Autodesk Fusion 360 part; units mm, degrees
sketch "Sketch1" plane through (0, 0, 0) normal (0, 1, 0) x (1, 0, 0)
  circle A0 centre (0, 0) radius 11
  circle A1 centre (0, 0) radius 12.5
  line L0 (0, 0) -> (9.5756, 8.0348)
  line L1 (0, 0) -> (12.5, 0) construction
  line L2 (0, 0) -> (-9.5756, 8.0348)
  line L3 (0, 0) -> (12.5, 0) construction
  line L4 (0, 0) -> (-4.7878, 11.5467)
  line L5 (-4.7878, 11.5467) -> (4.7878, 11.5467)
  circle A2 centre (0, 11.5467) radius 4.8552
  line L6 (0, 11.5467) -> (0, 16.402)
  circle A3 centre (0, 13.9744) radius 1.05
  circle A4 centre (0, 13.9744) radius 0.5
  line L7 (0, 16.402) -> (-0.6, 16.402)
  line L8 (0, 16.402) -> (0.6, 16.402)
  line L9 (-0.6, 16.402) -> (-0.6, 14.836)
  line L10 (0.6, 16.402) -> (0.6, 14.836)
  line L11 (0, 0) -> (6.25, 10.8253)
  line L12 (0, 0) -> (12.5, 0) construction
  line L13 (0, 0) -> (-6.25, 10.8253)
  line L14 (0, 11.5467) -> (2, 11.5467)
  line L15 (0, 11.5467) -> (-2, 11.5467)
  line L16 (2, 11.5467) -> (-2, 11.5467)
  line L17 (-2, 11.5467) -> (-2, 15.9709)
  line L18 (-2, 15.9709) -> (2, 15.9709)
  line L19 (2, 15.9709) -> (2, 11.5467)
  dimension "d1" = 22
  dimension "d2" = 25
  dimension "d3" = 40
  dimension "d4" = 140
  dimension "d5" = 2.1
  dimension "d6" = 1
  dimension "d7" = 0.6
  dimension "d8" = 0.6
  dimension "d9" = 60
  dimension "d10" = 120
  dimension "d13" = 2
  dimension "d14" = 2
  dimension "d15" = 9.5756
  dimension "d16" = 4.4242
extrude "Extrude1" add sketch "Sketch1" along normal blind 12 contours A0 A1 A2 L11 | A0 A1 A2 L13 | A0 A1 L4 L5 A2 L14 L15 L16 | A0 A1 L4 A2 | A1 L5 L17 | A1 L5 L19 | A1 L6 A3 L9 L17 L18 | A2 L9 L18 | A1 L5 L6 L15 L16 L17 | A1 L5 L6 L14 L16 L19 | A1 L6 A3 L10 L18 L19 | A2 L10 L18
sketch "Sketch2" plane through (0, 0, 0) normal (0, -1, 0) x (1, 0, 0)
  line L0 (0.6, -14.836) -> (0.6, -16.3648)
  arc A0 (0.6, -16.3648) -> (2, -15.9709) centre (0, -11.5467) ccw
  line L1 (2, -15.9709) -> (2, -12.339)
  arc A1 (2, -12.339) -> (6.25, -10.8253) centre (0, 0) ccw
  line L2 (6.25, -10.8253) -> (5.5, -9.5263)
  arc A2 (-5.5, -9.5263) -> (5.5, -9.5263) centre (0, 0) ccw
  line L3 (-5.5, -9.5263) -> (-6.25, -10.8253)
  arc A3 (-6.25, -10.8253) -> (-2, -12.339) centre (0, 0) ccw
  line L4 (-2, -12.339) -> (-2, -15.9709)
  arc A4 (-2, -15.9709) -> (-0.6, -16.3648) centre (0, -11.5467) ccw
  line L5 (-0.6, -16.3648) -> (-0.6, -14.836)
  arc A5 (0.6, -14.836) -> (-0.6, -14.836) centre (0, -13.9744) ccw
  line L6 (0, -11) -> (0, -12.9244)
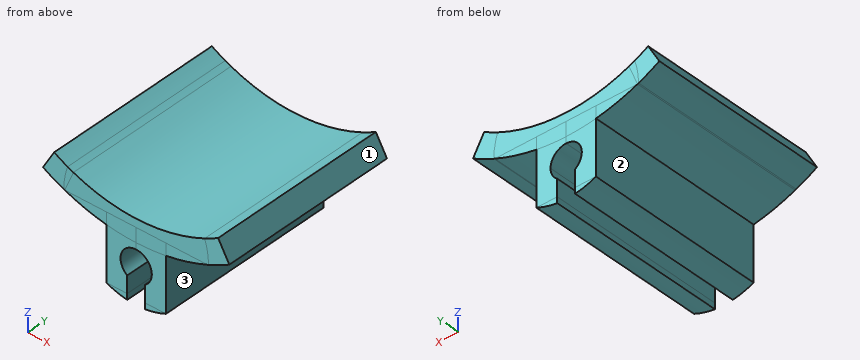
Verification items for the finished model (mm, model axes). Face numbers are marked on the shaded views. A direction names the side the tool comes from. Coordinates: 2 decimals unless noted, no trailing zeros. Write each loop counter-clockwise with the first axis right and the second up, starting at its lowest first coordinate (ties: lowest second). Pieces come first, ordered by that corner, then holes. Notation, with made-up numbers: M 49.25,60 L 103.25,60 A29 cw 103.25,93 Z; hole C 37,-18.75 d7. An arc over 180 degrees is marked long. One line per item, written item: value.
Item 1: Gauge pin test, flat ends, axial feed: pin 1 Ø1.1 at (y, z) = (5, -14.5) entering from -X; pin 2 Ø3 at (y, z) = (3, -14.5) entering from +X; pin 3 Ø3 at (x, y) = (3.5, 6.5) entering from +Z. Record the tip position at first contact, or that the pin passes through.
Check sheet entries:
pin 1: stops at x = -2
pin 2: stops at x = 2
pin 3: stops at z = -9.8
Item 2: Section check D-D, the plane x = -1.5. Record the boundary of the cut face in (y, z), plus the area to 3 significant figures.
Check sheet entries:
outline: M 0,-16.16 L 12,-16.16 L 12,-10.9 L 0,-10.9 Z
area: 63.2 mm^2
Item 3: Scan lines: line 1 along X through (y, z) = (11.25, -14); line 2 along X through (y, z) = (1, -15.75); line 3 along Z through (x, y) = (1.75, 8.75). Record each from-to range of solid material in increasing order.
Check sheet entries:
line 1: x = -2 to -1.05, 1.05 to 2
line 2: x = -2 to -0.6, 0.6 to 2
line 3: z = -16.08 to -10.86
Item 4: Section check A-A, the plane z = -15.25. Record the boundary of the cut face in (x, y), plus the area to 3 significant figures.
Check sheet entries:
outline: M -2,0 L -0.6,0 L -0.6,12 L -2,12 Z; M 0.6,0 L 2,0 L 2,12 L 0.6,12 Z
area: 33.6 mm^2
Item 5: Section check C-C, the plane z = -13.5. Record the boundary of the cut face in (x, y), plus the area to 3 significant figures.
Check sheet entries:
outline: M -2,0 L -0.94,0 L -0.94,12 L -2,12 Z; M 0.94,0 L 2,0 L 2,12 L 0.94,12 Z
area: 25.5 mm^2
Item 6: Section check B-B, the plane y = 1.75. Record the boundary of the cut face in (x, z), plus the area to 3 significant figures.
Check sheet entries:
outline: M -6.25,-10.83 A12.5 ccw -2,-12.34 L -2,-15.97 A4.86 ccw -0.6,-16.36 L -0.6,-14.84 A1.05 cw long 0.6,-14.84 L 0.6,-16.36 A4.86 ccw 2,-15.97 L 2,-12.34 A12.5 ccw 6.25,-10.83 L 5.5,-9.53 A11 cw -5.5,-9.53 Z
area: 28.5 mm^2
Item 7: Access from +Z, -Z, +X, -X, +Y, -Y to the whole of each face (thin tool, end or side, straight path). Record for the marked faces 1, 2 and 3.
Check sheet entries:
face 1: +Z, +X, +Y, -Y
face 2: -Z, -X, +Y, -Y
face 3: -Z, +X, +Y, -Y
